Drawing for the job (mm, zero at the part's lowest x, y, z). A direction names the side the tool comes from. Give positions to 0.01 mm unless a question says otherwise; leave off trailing zeros. Write each loop counter-clockwise with the first axis right and the second up, starting at its lowest first coordinate (ties: lowest second). Pieces come first, ordered by that corner, then holes.
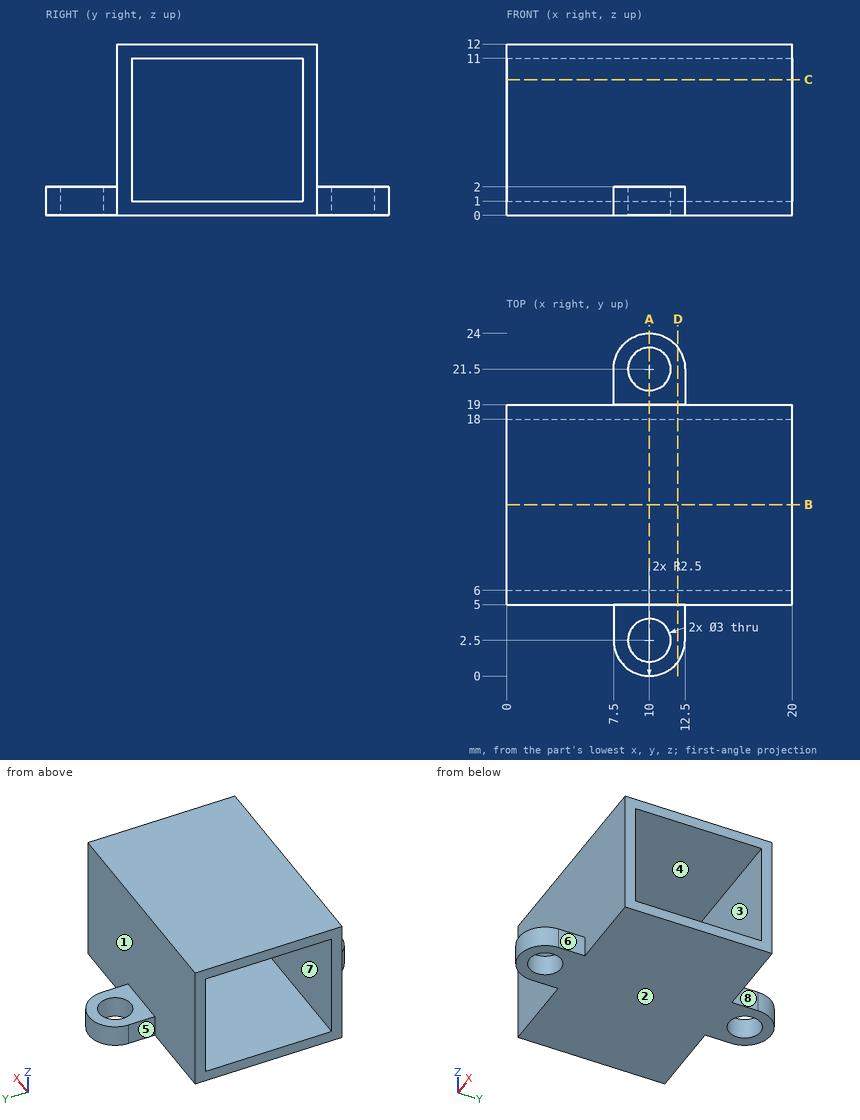
1. Slice it at D-D, the plane x = 12. Write the cut outline in (y, z), and give its area (3 significant figures).
Calculated:
outline: (1, 0) - (23, 0) - (23, 2) - (19, 2) - (19, 12) - (5, 12) - (5, 2) - (1, 2) - close; hole (6, 1) - (18, 1) - (18, 11) - (6, 11) - close
area: 64.0 mm2
2. Pin check, flat tips, straight feed: P1, Ø1, axis at y = 3.5, z = 1.5, coming from the -X side; P2, Ø4, axis at x = 12.5, z = 4.5, coming from the -Y side; P3, Ø5, axis at x = 5, z = 6.5, coming from the +Y side; P4, Ø1.8, axis at x = 10, y = 21.5, coming from the +Z side. Stop position of each tip, or through.
Calculated:
P1: stops at x = 7.5
P2: stops at y = 5
P3: stops at y = 19
P4: passes through
3. Slice it at C-C, the plane z = 9.5. Write the cut outline in (x, y).
Calculated:
outline: (0, 5) - (20, 5) - (20, 6) - (0, 6) - close; (0, 18) - (20, 18) - (20, 19) - (0, 19) - close
4. Which spindle directions (+Z, -Z, +X, -X, +Y, -Y) get a long thin tool onto all of the face, cutting with end or side? Do the marked faces 5, 6, 7 and 8. Say none if no direction does.
Calculated:
face 5: +Z, -Z, -X, +Y
face 6: +Z, -Z, +X, -Y
face 7: +X, -X
face 8: +Z, -Z, +X, +Y
5. Slice it at B-B, the plane y = 12. Write the cut outline in (x, z), and give its area (3 significant figures).
Calculated:
outline: (0, 0) - (20, 0) - (20, 1) - (0, 1) - close; (0, 11) - (20, 11) - (20, 12) - (0, 12) - close
area: 40.0 mm2
6. Probe probe 1 along Y at (x, z) = (10, 0.8); probe 2 along Y at (x, z) = (10, 1.2); probe 3 along Z at (x, y) = (18, 16.5). List the from-to ranges inside material, lowest first.
Calculated:
probe 1: y = 0 to 1, 4 to 20, 23 to 24
probe 2: y = 0 to 1, 4 to 6, 18 to 20, 23 to 24
probe 3: z = 0 to 1, 11 to 12
7. Pull direction Z, two halves, no side cores. Call the marked faces 1, 2, 3 and 4: +Z half, -Z half, draft (parallel to the pull), parting line (faces both ways), or undercut.
Calculated:
face 1: draft
face 2: -Z half
face 3: undercut
face 4: undercut
8. Slice it at A-A, the plane x = 10. Write the cut outline in (y, z).
Calculated:
outline: (0, 0) - (1, 0) - (1, 2) - (0, 2) - close; (4, 0) - (20, 0) - (20, 2) - (19, 2) - (19, 12) - (5, 12) - (5, 2) - (4, 2) - close; (23, 0) - (24, 0) - (24, 2) - (23, 2) - close; hole (6, 1) - (18, 1) - (18, 11) - (6, 11) - close
